Source: CAD feature listing. Evaluate the final solid. Frame: model axes, mm. A direction names the side the tool comes from. Give positions to 0.01 mm unless a question says otherwise; leave off trailing zeros. Write each loop counter-clockwise with the first axis right and the second up, starting at its lowest first coordinate (ties: lowest second). Pieces come first, ordered by that corner, then holes. Notation, with made-up numbers: (56.5, 57.25) -> (91.5, 57.25) arc R16 ccw to (91.5, 62.25) -> close; hole circle Ø2 at (-32.5, 39). An arc over 180 degrees is marked (long way). Write item = value, one per line.
from build123d import *

# Parameters (mm, degrees)
F1_DEPTH = 80
F3_R     = 3.05
F4_DEPTH = 25
F2_R     = 2.5
F2_R_2   = 20
F5_DEPTH = 4


with BuildPart() as f1:
    # F0 (on Front) → F1 (new body)
    with BuildSketch(Plane.XZ):
        Polygon((0, 60), (0, 0), (60, 0), (60, 4), (4, 4), (4, 60), align=None)
    extrude(amount=F1_DEPTH)

    # F3 (on face) → F4 (cut)
    with BuildSketch(Plane(origin=(0, 0, 0), x_dir=(1, 0, 0), z_dir=(0, 0, -1))):
        with Locations((25, 73)):
            Circle(F3_R)
        with Locations((25, 7)):
            Circle(F3_R)
    extrude(amount=-F4_DEPTH, mode=Mode.SUBTRACT)

    # F2 (on face) → F5 (cut, through all)
    with BuildSketch(Plane(origin=(0, 0, 0), x_dir=(0, -1, 0), z_dir=(-1, 0, 0))):
        with Locations((16.43, 56.57)):
            Circle(F2_R)
        with Locations((40, 33)):
            Circle(F2_R_2)
        with Locations((63.57, 56.57)):
            Circle(F2_R)
        with Locations((16.43, 9.43)):
            Circle(F2_R)
        with Locations((63.57, 9.43)):
            Circle(F2_R)
    extrude(amount=-F5_DEPTH, mode=Mode.SUBTRACT)


solid = f1.part
1) Cut plane C-C (z = 9.43). Return the cut outline in (x, y), then the cut area to 3 significant figures.
Computed:
outline = (0, -80) -> (4, -80) -> (4, -66.07) -> (0, -66.07) -> close; (0, -61.07) -> (4, -61.07) -> (4, -18.93) -> (0, -18.93) -> close; (0, -13.93) -> (4, -13.93) -> (4, 0) -> (0, 0) -> close
area = 280 mm²
2) Draft query along Y for faces 3 (the flat face through (4, -31, 13)), 4 (the cylindrical face through (1.972, -61.072, 9.54)), 5 (the flat face through (3, -80, 17)). Return one class per face: pulls with the +Y half, pulls with the -Y half, needs draft (parallel to the pull), parting line crosses it, or undercut.
Computed:
face_3 = needs draft
face_4 = undercut
face_5 = pulls with the -Y half
3) Cut plane A-A (y = -63.57). Return the cut outline in (x, z), then the cut area to 3 significant figures.
Computed:
outline = (0, 0) -> (60, 0) -> (60, 4) -> (4, 4) -> (4, 6.93) -> (0, 6.93) -> close; (0, 11.93) -> (4, 11.93) -> (4, 54.07) -> (0, 54.07) -> close; (0, 59.07) -> (4, 59.07) -> (4, 60) -> (0, 60) -> close
area = 424 mm²
4) Cut plane D-D (z = 33). Return the cut outline in (x, y), then the cut area to 3 significant figures.
Computed:
outline = (0, -80) -> (4, -80) -> (4, -60) -> (0, -60) -> close; (0, -20) -> (4, -20) -> (4, 0) -> (0, 0) -> close
area = 160 mm²
5) Cut plane B-B (y = -73). Return the cut outline in (x, z), then the cut area to 3 significant figures.
Computed:
outline = (0, 0) -> (21.95, 0) -> (21.95, 4) -> (4, 4) -> (4, 60) -> (0, 60) -> close; (28.05, 0) -> (60, 0) -> (60, 4) -> (28.05, 4) -> close
area = 440 mm²
6) Access query for faces 1 (the flat face through (32, -39, 4)), 2 (the cylindrical face through (1.97, -17.77, 58.68)). Directions: +Z, -Z, +X, -X, +Y, -Y. A direction counts if a zero-diameter tool reaches every point of the face in a straight line with its end or side. Return the directions, or none.
Computed:
face_1 = +Z, +X, +Y, -Y
face_2 = +X, -X
7) Contact query for flat-ended pins moving along their axis: pin 1 (3 mm diameter, centred on y = -63.57, z = 56.57, fed in from +X); pin 2 (17 mm diameter, centred on x = 19.5, y = -42, fed in from +Z). Output: stop coordinate, or through.
Computed:
pin_1 = through
pin_2 = 4
8) Material intervals for L1, parallel to Z at x = 1.4, y = -16.43; L2, parallel to Y at x = 25, z = 1.1; L3, parallel to Y at x = 2, z = 56, sorted ascending.
Computed:
L1 = 0 to 6.93, 11.93 to 54.07, 59.07 to 60
L2 = -80 to -76.05, -69.95 to -10.05, -3.95 to 0
L3 = -80 to -66, -61.14 to -18.86, -14 to 0
